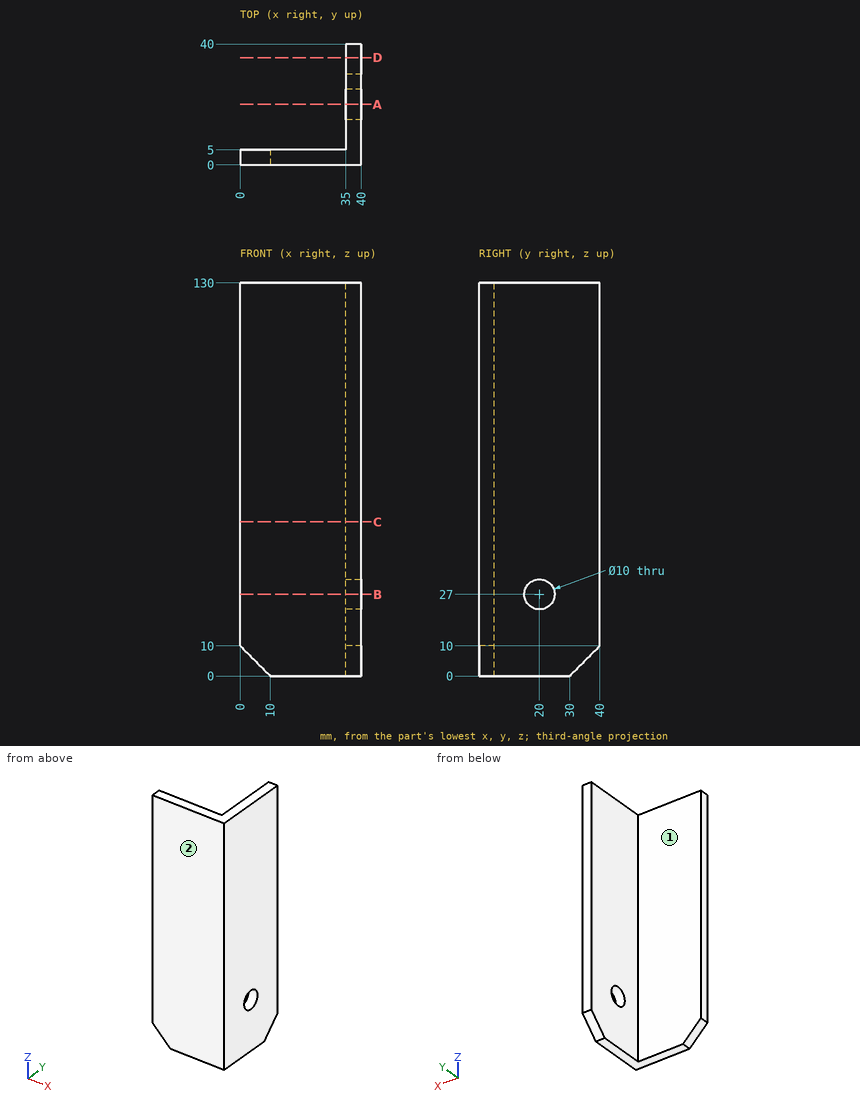
Could you check a few things on this drawing? It's one solid part, dimensions in mm from its lowest x, y, z. A direction names the side the tool comes from. Give positions to 0.01 mm unless a question says otherwise; leave off trailing zeros. Order: outer loops, then holes, each group sorted by start corner. A loop starts at its lowest first (then second) coordinate and runs counter-clockwise, first axis right, second up. Notation, with made-up numbers: M -14,-27 L -1,-27 A24 ccw -1,-16 Z; hole C 65,1.5 d6. An arc over 180 degrees is marked long. Use one line per item in the form item = value. Start each with the question number.
Item 1: If we section it at A-A (y = 20): Write out the boundary of the cut face in (x, z), then the cut area to 3 significant figures.
Item 2: If we section it at B-B (z = 27): Write out the boundary of the cut face in (x, y), then the cut area to 3 significant figures.
Item 3: For the marked faces 1 and 2, which set-ups out of +Z, -Z, +X, -X, +Y, -Y let a thin tool reach every point of the face, with its end or its side?
Item 4: If we section it at D-D (y = 35.5): Write out the boundary of the cut face in (x, z).
Item 5: Will these pins go through, and if not, where does the flat tip stop? pin 1 Ø10.5 at (y, z) = (26, 66) entering from -X; pin 2 Ø3 at (x, z) = (15, 31) entering from +Y; pin 3 Ø10 at (x, y) = (19.5, 13.5) entering from +Z.
Item 6: If we section it at C-C (z = 51): Write out the boundary of the cut face in (x, y).
Item 7: If I drill on line 1 along Y through (x, z) = (37.45, 27); line 2 along X through (y, z) = (32.5, 101); line 3 along Y through (x, z) = (14, 91.5), over which ranges is the centre line in solid material (lowest first)?
Outcome:
q1.outline = M 35,0 L 40,0 L 40,22 L 35,22 Z; M 35,32 L 40,32 L 40,130 L 35,130 Z
q1.area = 600 mm2
q2.outline = M 0,0 L 40,0 L 40,15 L 35,15 L 35,5 L 0,5 Z; M 35,25 L 40,25 L 40,40 L 35,40 Z
q2.area = 325 mm2
q3.face_1 = +Z, -Z, -X, +Y
q3.face_2 = +Z, -Z, +X, -X, -Y
q4.outline = M 35,5.5 L 40,5.5 L 40,130 L 35,130 Z
q5.pin_1 = 35
q5.pin_2 = 5
q5.pin_3 = through
q6.outline = M 0,0 L 40,0 L 40,40 L 35,40 L 35,5 L 0,5 Z
q7.line_1 = 0 to 15, 25 to 40
q7.line_2 = 35 to 40
q7.line_3 = 0 to 5
